```python
from build123d import *

# Parameters (mm, degrees)
SKETCH_1_W          = 43
SKETCH_1_H          = 110
SKETCH_1_W_2        = 21.5
SKETCH_1_H_2        = 15
SKETCH_1_R          = 2.5
EXTRUDE_1_DEPTH     = 9
SKETCH_4_R          = 15
EXTRUDE_2_DEPTH     = 5
SKETCH_5_W          = 220.601907976
SKETCH_5_H          = 5
EXTRUDE_3_DEPTH     = 28
SKETCH_6_R          = 15
CUT_EXTRUDE_1_DEPTH = 28


with BuildPart() as part:
    # 草图1 → 凸台-拉伸1 (new body)
    # profile 1 of 3: a face of its own
    with BuildSketch(Plane.XY):
        with Locations((0.290540541, -64.442567568)):
            Rectangle(SKETCH_1_W, SKETCH_1_H)
    # profile 2 of 3: a face of its own
    with BuildSketch(Plane.XY):
        with Locations((11.040540541, -1.942567568)):
            Rectangle(SKETCH_1_W_2, SKETCH_1_H_2)
        with Locations((12.790540541, -1.442567568)):
            Circle(SKETCH_1_R, mode=Mode.SUBTRACT)
    # profile 3 of 3: a face of its own
    with BuildSketch(Plane.XY):
        with Locations((-10.459459459, -1.942567568)):
            Rectangle(SKETCH_1_W_2, SKETCH_1_H_2)
        with Locations((-12.209459459, -1.442567568)):
            Circle(SKETCH_1_R, mode=Mode.SUBTRACT)
    extrude(amount=EXTRUDE_1_DEPTH)

    # 草图4 → 凸台-拉伸2 (add)
    with BuildSketch(Plane.XY.offset(9)):
        with Locations(Location((0, -104.442567568, 0), (0, 0, 270))):
            Circle(SKETCH_4_R)
    extrude(amount=EXTRUDE_2_DEPTH)

    # 草图5 → 凸台-拉伸3 (add)
    with BuildSketch(Plane.XY.offset(14)):
        with Locations((0, -104.442567568)):
            Rectangle(SKETCH_5_W, SKETCH_5_H)
    extrude(amount=EXTRUDE_3_DEPTH)

    # 草图6 → 切除-拉伸1 (cut)
    with BuildSketch(Plane(origin=(0, -106.942567568, 0), x_dir=(-1, 0, 0), z_dir=(0, -1, 0))):
        with Locations((-19.127702363, -42)):
            Circle(SKETCH_6_R)
        with Locations((-54.127702363, -42)):
            Circle(SKETCH_6_R)
        with Locations((-89.127702363, -42)):
            Circle(SKETCH_6_R)
        with Locations((19.127702363, -42)):
            Circle(SKETCH_6_R)
        with Locations((54.127702363, -42)):
            Circle(SKETCH_6_R)
        with Locations((89.127702363, -42)):
            Circle(SKETCH_6_R)
    extrude(amount=-CUT_EXTRUDE_1_DEPTH, mode=Mode.SUBTRACT)


solid = part.part
```
Here's how the part is built. I have some questions about the finished solid (model axes, mm). A direction names the side the tool comes from. Give positions to 0.01 mm unless a question says otherwise; leave off trailing zeros. Write each loop counter-clockwise with the first axis right and the second up, starting at its lowest first coordinate (ties: lowest second). Pieces come first, ordered by that corner, then holes. Notation, with made-up numbers: (-4.75, 38) -> (28.25, 38) arc R12 cw to (28.25, 59) -> close; hole circle Ø1 at (17, 40.25). An arc over 180 degrees is marked (long way). Write each question's results on one line, items separated by ' | '.
Item 1: Suppose I cut it at B-B on x = -6.5. Write out the boundary of the cut face in (y, z).
Output:
outline: (-119.44, 0) -> (5.56, 0) -> (5.56, 9) -> (-90.92, 9) -> (-90.92, 14) -> (-101.94, 14) -> (-101.94, 33.9) -> (-106.94, 33.9) -> (-106.94, 14) -> (-117.96, 14) -> (-117.96, 9) -> (-119.44, 9) -> close
Item 2: On a 3-axis mill with a long thin cutter (end or side, diameter ignored), from which of +Z, -Z, +X, -X, +Y, -Y can I reach the whole of each face in a straight line? I mean faces 1 (the face through (-2, -106.943, 25)), 2 (the face through (107, -104, 42)), 3 (the face through (-2, -101.943, 25)). Say none if no direction works.
Output:
face 1: +Z, +X, -X, -Y | face 2: +Z, +X, -X, +Y, -Y | face 3: +Z, +X, -X, +Y
Item 3: Suppose I cut it at C-C on z = 4.5. Write out the boundary of the cut face in (x, y).
Output:
outline: (-21.21, -119.44) -> (21.79, -119.44) -> (21.79, 5.56) -> (-21.21, 5.56) -> close; hole circle Ø5 at (-12.21, -1.44); hole circle Ø5 at (12.79, -1.44)
Item 4: If I drill on L1, parallel to Y at x = 89, z = 26; L2, parallel to X at y = -10, z = 8.5; L3, parallel to Z at x = 12.5, y = -23, over which ranges is the centre line in solid material (lowest first)?
Output:
L1: y = -106.94 to -101.94 | L2: x = -21.21 to 21.79 | L3: z = 0 to 9
Item 5: Suppose I cut it at A-A on z = 36. Write out the boundary of the cut face in (x, y).
Output:
outline: (-110.3, -106.94) -> (-102.88, -106.94) -> (-102.88, -101.94) -> (-110.3, -101.94) -> close; (-75.38, -106.94) -> (-67.88, -106.94) -> (-67.88, -101.94) -> (-75.38, -101.94) -> close; (-40.38, -106.94) -> (-32.88, -106.94) -> (-32.88, -101.94) -> (-40.38, -101.94) -> close; (-5.38, -106.94) -> (5.38, -106.94) -> (5.38, -101.94) -> (-5.38, -101.94) -> close; (32.88, -106.94) -> (40.38, -106.94) -> (40.38, -101.94) -> (32.88, -101.94) -> close; (67.88, -106.94) -> (75.38, -106.94) -> (75.38, -101.94) -> (67.88, -101.94) -> close; (102.88, -106.94) -> (110.3, -106.94) -> (110.3, -101.94) -> (102.88, -101.94) -> close
Item 6: For pin 1 Ø4 at (x, y) = (-12.21, -1.44) entering from -Z; pin 2 Ø7 at (y, z) = (-77.5, 2.5) entering from +X; pin 3 Ø1 at (x, y) = (21, -84) entering from -Z; pin 4 Ø4.5 at (y, z) = (-79, 2.5) entering from -X, each with a flat end and sliding along its axis, tell me the tip position at first contact or that it passes through.
Output:
pin 1: passes through | pin 2: stops at x = 21.79 | pin 3: stops at z = 0 | pin 4: stops at x = -21.21
Item 7: Suppose I cut it at D-D on y = -38. Write out the boundary of the cut face in (x, z).
Output:
outline: (-21.21, 0) -> (21.79, 0) -> (21.79, 9) -> (-21.21, 9) -> close
